Source: CAD feature listing. Evaluate the final solid. Frame: model axes, mm. A direction names the side the tool comes from. Give positions to 0.01 mm unless a question says otherwise; leave off trailing zeros. Loops run counter-clockwise (first coordinate to the right, second up) from the corner with the lowest first, then second, coordinate; pieces in that order, holes last.
Autodesk Inventor part; units mm, degrees
ref_plane "cp_right_body_pole1_XY" through (4.8006, 0.3048, 3.3655) normal (0, -1, 0) x (1, 0, 0)
ref_plane "cp_right_body_pole1_YZ" through (4.8006, 0.3048, 3.3655) normal (1, 0, 0) x (0, 0, 1)
ref_plane "cp_right_body_pole1_ZX" through (4.8006, 0.3048, 3.3655) normal (0, 0, 1) x (0, -1, 0)
sketch "Sketch_1" plane through (0, 0, 0) normal (0, 0, 1) x (1, 0, 0)
  arc A0 (0, 0.1524) -> (0.1524, 0) centre (0.1524, 0.1524) ccw
  line L0 (0.1524, 0) -> (9.4488, 0)
  arc A1 (9.4488, 0) -> (9.6012, 0.1524) centre (9.4488, 0.1524) ccw
  line L1 (9.6012, 0.1524) -> (9.6012, 5.3848)
  line L2 (9.6012, 5.3848) -> (9.2964, 5.3848)
  line L3 (9.2964, 5.3848) -> (9.2964, 0.4572)
  arc A2 (9.144, 0.3048) -> (9.2964, 0.4572) centre (9.144, 0.4572) ccw
  line L4 (9.144, 0.3048) -> (0.4572, 0.3048)
  arc A3 (0.3048, 0.4572) -> (0.4572, 0.3048) centre (0.4572, 0.4572) ccw
  line L5 (0.3048, 0.4572) -> (0.3048, 5.3848)
  line L6 (0.3048, 5.3848) -> (0, 5.3848)
  line L7 (0, 5.3848) -> (0, 0.1524)
extrude "Extrusion1" add sketch "Sketch_1" along normal blind 5.334
sketch "Sketch_3" plane through (0, 0, 2.3622) normal (0, 0, 1) x (1, 0, 0)
  arc A0 (2.1031, -1.0313) -> (2.1031, -2.5501) centre (4.4075, -1.7907) ccw
  arc A1 (2.1082, -2.5819) -> (2.1031, -2.5501) centre (2.0066, -2.5819) ccw
  line L0 (2.1082, -2.5819) -> (2.1082, -3.5814)
  line L1 (2.1082, -3.5814) -> (2.413, -3.5814)
  line L2 (2.413, -3.5814) -> (2.413, -2.5819)
  arc A2 (2.413, -2.5819) -> (2.4079, -2.5501) centre (2.3114, -2.5819) ccw
  arc A3 (2.4079, -1.0313) -> (2.4079, -2.5501) centre (4.7123, -1.7907) ccw
  arc A4 (2.4079, -1.0313) -> (2.413, -0.9995) centre (2.3114, -0.9995) ccw
  line L3 (2.413, -0.9995) -> (2.413, 0)
  line L4 (2.413, 0) -> (2.1082, 0)
  line L5 (2.1082, 0) -> (2.1082, -0.9995)
  arc A5 (2.1031, -1.0313) -> (2.1082, -0.9995) centre (2.0066, -0.9995) ccw
extrude "Extrusion2" add sketch "Sketch_3" along normal blind 0.7112
sketch "Sketch_4" plane through (0, 0, 2.3622) normal (0, 0, 1) x (1, 0, 0)
  arc A0 (7.1882, -0.9995) -> (7.1933, -1.0313) centre (7.2898, -0.9995) ccw
  arc A1 (7.1933, -2.5501) -> (7.1933, -1.0313) centre (4.8889, -1.7907) ccw
  arc A2 (7.1933, -2.5501) -> (7.1882, -2.5819) centre (7.2898, -2.5819) ccw
  line L0 (7.1882, -2.5819) -> (7.1882, -3.5814)
  line L1 (7.1882, -3.5814) -> (7.493, -3.5814)
  line L2 (7.493, -3.5814) -> (7.493, -2.5819)
  arc A3 (7.4981, -2.5501) -> (7.493, -2.5819) centre (7.5946, -2.5819) ccw
  arc A4 (7.4981, -2.5501) -> (7.4981, -1.0313) centre (5.1937, -1.7907) ccw
  arc A5 (7.493, -0.9995) -> (7.4981, -1.0313) centre (7.5946, -0.9995) ccw
  line L3 (7.493, -0.9995) -> (7.493, 0)
  line L4 (7.493, 0) -> (7.1882, 0)
  line L5 (7.1882, 0) -> (7.1882, -0.9995)
extrude "Extrusion3" add sketch "Sketch_4" along normal blind 0.7112
sketch "Sketch_5" plane through (0, 0, 0) normal (1, 0, 0) x (0, 1, 0)
  line L0 (-3.3274, 3.0734) -> (-3.8354, 3.0734)
  line L1 (-3.8354, 3.0734) -> (-3.8354, 2.3622)
  line L2 (-3.8354, 2.3622) -> (-3.3274, 2.3622)
  arc A0 (-3.3274, 3.0734) -> (-3.3274, 2.3622) centre (-3.2408, 2.7178) ccw
extrude "Extrusion4" cut sketch "Sketch_5" along normal blind 8.3058
sketch "Sketch_6" plane through (0, 0, 0) normal (1, 0, 0) x (0, 1, 0)
  line L0 (2.8448, 3.3655) -> (2.8448, 1.3335)
  line L1 (2.8448, 1.3335) -> (4.3688, 1.3335)
  line L2 (4.3688, 1.3335) -> (4.3688, 3.3655)
  line L3 (4.3688, 3.3655) -> (2.8448, 3.3655)
extrude "Extrusion5" cut sketch "Sketch_6" along normal blind 10.16
sketch "Sketch_7" plane through (0, 0, 0) normal (1, 0, 0) x (0, 1, 0)
  line L0 (1.651, 3.4449) -> (0, 3.4449)
  line L1 (0, 3.4449) -> (0, 1.9209)
  line L2 (0, 1.9209) -> (1.651, 1.9209)
  arc A0 (1.651, 1.9209) -> (1.651, 3.4449) centre (1.0795, 2.6829) ccw
extrude "Extrusion6" cut sketch "Sketch_7" along normal blind 0.3048
sketch "Sketch_8" plane through (9.8044, 0, 0) normal (1, 0, 0) x (0, 0, -1)
  line L0 (-3.4449, 1.651) -> (-3.4449, 0)
  line L1 (-3.4449, 0) -> (-1.9209, 0)
  line L2 (-1.9209, 0) -> (-1.9209, 1.651)
  arc A0 (-1.9209, 1.651) -> (-3.4449, 1.651) centre (-2.6829, 1.0795) ccw
extrude "Extrusion7" cut sketch "Sketch_8" against normal blind 0.508
sketch "Sketch_9" plane through (0, 0, 0) normal (0, 1, 0) x (-1, 0, 0)
  line L0 (0, 1.9209) -> (0, 3.4449)
  line L1 (0, 3.4449) -> (-1.143, 3.4449)
  arc A0 (-1.143, 3.4449) -> (-1.143, 1.9209) centre (-0.5715, 2.6829) ccw
  line L2 (-1.143, 1.9209) -> (0, 1.9209)
extrude "Extrusion8" cut sketch "Sketch_9" along normal blind 0.508
sketch "Sketch_10" plane through (0, 0, 0) normal (0, 1, 0) x (-1, 0, 0)
  arc A0 (-8.6614, 1.9209) -> (-8.6614, 3.4449) centre (-9.2329, 2.6829) ccw
  line L0 (-8.6614, 3.4449) -> (-9.8044, 3.4449)
  line L1 (-9.8044, 3.4449) -> (-9.8044, 1.9209)
  line L2 (-9.8044, 1.9209) -> (-8.6614, 1.9209)
extrude "Extrusion9" cut sketch "Sketch_10" along normal blind 0.508
sketch "Sketch_11" plane through (0.3048, 0, 0) normal (1, 0, 0) x (0, 0, -1)
  line L0 (0, -0.4826) -> (0.3048, -0.4826)
  line L1 (0.3048, -0.4826) -> (0.3048, 0.1778)
  arc A0 (0.3048, 0.1778) -> (0.1778, 0.3048) centre (0.1778, 0.1778) ccw
  line L2 (0.1778, 0.3048) -> (0, 0.3048)
  line L3 (0, 0.3048) -> (0, -0.4826)
extrude "Extrusion10" add sketch "Sketch_11" along normal blind 0.508
sketch "Sketch_12" plane through (9.2964, 0, 0) normal (1, 0, 0) x (0, 0, -1)
  line L0 (0, -0.4826) -> (0.3048, -0.4826)
  line L1 (0.3048, -0.4826) -> (0.3048, 0.1778)
  arc A0 (0.3048, 0.1778) -> (0.1778, 0.3048) centre (0.1778, 0.1778) ccw
  line L2 (0.1778, 0.3048) -> (0, 0.3048)
  line L3 (0, 0.3048) -> (0, -0.4826)
extrude "Extrusion11" add sketch "Sketch_12" against normal blind 0.508
sketch "Sketch_13" plane through (4.8006, 0, 0) normal (1, 0, 0) x (0, 0, -1)
  line L0 (-5.6388, -0.4826) -> (-5.334, -0.4826)
  line L1 (-5.334, -0.4826) -> (-5.334, 0.3048)
  line L2 (-5.334, 0.3048) -> (-5.5118, 0.3048)
  arc A0 (-5.5118, 0.3048) -> (-5.6388, 0.1778) centre (-5.5118, 0.1778) ccw
  line L3 (-5.6388, 0.1778) -> (-5.6388, -0.4826)
extrude "Extrusion12" add sketch "Sketch_13" along normal blind 0.508
ref_plane "cp_right_body_pole1_XY" through (4.8006, 0.3048, 3.3655) normal (0, -1, 0) x (1, 0, 0)
ref_plane "cp_right_body_pole1_YZ" through (4.8006, 0.3048, 3.3655) normal (1, 0, 0) x (0, 0, 1)
ref_plane "cp_right_body_pole1_ZX" through (4.8006, 0.3048, 3.3655) normal (0, 0, 1) x (0, -1, 0)
properties part number "AS11CHra1"
1) Ray query, probe 1 along X at (y, z) = (4, 0.9); probe 2 along X at (y, z) = (-0.5, 3); probe 3 along Y at (x, z) = (2.5, 3.55). Return the intervals inside material, ascending.
Checks:
probe 1: x = 0 to 0.3, 9.3 to 9.6
probe 2: x = 2.11 to 2.41, 7.19 to 7.49
probe 3: y = 0 to 0.3
2) Reachability of faces 1 (the flat face through (0, 2.2, 2.6)), 2 (the flat face through (9.45, 0.63, 1.921)), 3 (the flat face through (0.18, 0.26, 1.921)), 4 (the flat face through (9.296, 2.4, 2.6)) from +Z, -Z, +X, -X, +Y, -Y: full face, straight path, thin tool, end or side. Return the list, or none.
Checks:
face 1: +Z, -Z, -X, +Y, -Y
face 2: +X, -Y
face 3: -X, -Y
face 4: +Z, -Z, +Y
3) Cut plane C-C (y = 5.25). Return loops of the section in (x, z).
Checks:
outline: (0, 0) - (0.3, 0) - (0.3, 5.33) - (0, 5.33) - close; (9.3, 0) - (9.6, 0) - (9.6, 5.33) - (9.3, 5.33) - close
4) Contact query for flat-ended pins moving along their axis: P1, Ø0.8, axis at x = 9, y = 1, coming from the +Z side; P2, Ø3, axis at x = 5, z = 4.5, coming from the -Y side; P3, Ø1, axis at x = 4, z = 1.5, coming from the +Y side. Output: stop coordinate, or through.
Checks:
P1: stops at z = 5.33
P2: stops at y = -0.48
P3: stops at y = 0.3
5) Cut plane D-D (z = 5.2). Return loops of the section in (x, y).
Checks:
outline: (0, 0.15) arc R0.15 ccw to (0.15, 0) - (9.45, 0) arc R0.15 ccw to (9.6, 0.15) - (9.6, 5.38) - (9.3, 5.38) - (9.3, 0.46) arc R0.15 cw to (9.14, 0.3) - (0.46, 0.3) arc R0.15 cw to (0.3, 0.46) - (0.3, 5.38) - (0, 5.38) - close
6) Pull-direction query (X, two-part tool) for faces 5 (the flat face through (0.18, 0.29, 3.445)), 6 (the flat face through (0.305, 2.3, 2.6)), 7 (the flat face through (9.601, 2.2, 2.6)), 8 (the flat face through (5, 0.305, 3)); classes: released by +X, released by -X, zero draft, split by the parting line, or undercut.
Checks:
face 5: zero draft
face 6: undercut
face 7: released by +X
face 8: undercut
7) Cut plane B-B (z = 1.7). Return loops of the section in (x, y).
Checks:
outline: (0, 0.15) arc R0.15 ccw to (0.15, 0) - (9.45, 0) arc R0.15 ccw to (9.6, 0.15) - (9.6, 2.84) - (9.3, 2.84) - (9.3, 0.46) arc R0.15 cw to (9.14, 0.3) - (0.46, 0.3) arc R0.15 cw to (0.3, 0.46) - (0.3, 2.84) - (0, 2.84) - close; (0, 4.37) - (0.3, 4.37) - (0.3, 5.38) - (0, 5.38) - close; (9.3, 4.37) - (9.6, 4.37) - (9.6, 5.38) - (9.3, 5.38) - close
8) Cut plane A-A (y = 4.25). Return loops of the section in (x, z).
Checks:
outline: (0, 0) - (0.3, 0) - (0.3, 1.33) - (0, 1.33) - close; (0, 3.37) - (0.3, 3.37) - (0.3, 5.33) - (0, 5.33) - close; (9.3, 0) - (9.6, 0) - (9.6, 1.33) - (9.3, 1.33) - close; (9.3, 3.37) - (9.6, 3.37) - (9.6, 5.33) - (9.3, 5.33) - close
